Source: CAD feature listing. Evaluate the final solid. Frame: model axes, mm. Give positions to 0.01 mm unless a question says otherwise; leave off trailing zeros. Order: outer loops, then holes, each group sorted by start corner. A loop starts at its lowest first (then second) coordinate and runs counter-clockwise, first axis right, second up.
from build123d import *

# Parameters (mm, degrees)
F1_DEPTH = 0.8
F3_DEPTH = 25


# Not quite as in the source:
# - a feature names something its author has since deleted; it is built from what else it names


with BuildPart() as f1:
    # F0 (on Front) → F1 (new body, symmetric)
    with BuildSketch(Plane.XZ):
        Polygon((609, -150), (609, 150), (-609, 150), (-609, -150), (-98.2216194272, -150), (-98.2216194272, -80), (101.7783805728, -80), (101.7783805728, -150), align=None)
    extrude(amount=F1_DEPTH, both=True)

    # F2 (on face) → F3 (cut)
    with BuildSketch(Plane.XZ.offset(0.8)):
        with BuildLine():
            Line((-609, 0), (-586.7130714899, 0))
            ThreePointArc((-586.7130714899, 0), (-593.05140569, 16.7836636007), (-609, 25))
            Line((-609, 25), (-609, 0))
        make_face()
        with BuildLine():
            ThreePointArc((-460, 0), (-435, -25), (-410, 0))
            Line((-410, 0), (-435, 0))
            Line((-435, 0), (-460, 0))
        make_face()
        with BuildLine():
            Line((-435, 0), (-410, 0))
            ThreePointArc((-410, 0), (-435, 25), (-460, 0))
            Line((-460, 0), (-435, 0))
        make_face()
        with BuildLine():
            ThreePointArc((-286, 0), (-261, -25), (-236, 0))
            Line((-236, 0), (-261, 0))
            Line((-261, 0), (-286, 0))
        make_face()
        with BuildLine():
            Line((-261, 0), (-236, 0))
            ThreePointArc((-236, 0), (-261, 25), (-286, 0))
            Line((-286, 0), (-261, 0))
        make_face()
        with BuildLine():
            ThreePointArc((-112, 0), (-87, -25), (-62, 0))
            Line((-62, 0), (-87, 0))
            Line((-87, 0), (-112, 0))
        make_face()
        with BuildLine():
            Line((-87, 0), (-62, 0))
            ThreePointArc((-62, 0), (-87, 25), (-112, 0))
            Line((-112, 0), (-87, 0))
        make_face()
        with BuildLine():
            ThreePointArc((112, 0), (87, 25), (62, 0))
            Line((62, 0), (87, 0))
            Line((87, 0), (112, 0))
        make_face()
        with BuildLine():
            Line((87, 0), (62, 0))
            ThreePointArc((62, 0), (87, -25), (112, 0))
            Line((112, 0), (87, 0))
        make_face()
        with BuildLine():
            ThreePointArc((286, 0), (261, 25), (236, 0))
            Line((236, 0), (261, 0))
            Line((261, 0), (286, 0))
        make_face()
        with BuildLine():
            Line((261, 0), (236, 0))
            ThreePointArc((236, 0), (261, -25), (286, 0))
            Line((286, 0), (261, 0))
        make_face()
        with BuildLine():
            ThreePointArc((460, 0), (435, 25), (410, 0))
            Line((410, 0), (435, 0))
            Line((435, 0), (460, 0))
        make_face()
        with BuildLine():
            Line((435, 0), (410, 0))
            ThreePointArc((410, 0), (435, -25), (460, 0))
            Line((460, 0), (435, 0))
        make_face()
        with BuildLine():
            ThreePointArc((-609, -24.7047928188), (-593.1499526355, -16.5983450419), (-586.7130714899, 0))
            Line((-586.7130714899, 0), (-609, 0))
            Line((-609, 0), (-609, -24.7047928188))
        make_face()
        with BuildLine():
            ThreePointArc((609, 25), (591.3223304703, 17.6776695297), (584, 0))
            Line((584, 0), (609, 0))
            Line((609, 0), (609, 25))
        make_face()
        with BuildLine():
            Line((609, 0), (584, 0))
            ThreePointArc((584, 0), (591.3223304703, -17.6776695297), (609, -25))
            Line((609, -25), (609, 0))
        make_face()
        with BuildLine():
            ThreePointArc((-532, 0), (-522, -10), (-512, 0))
            Line((-512, 0), (-532, 0))
        make_face()
        with BuildLine():
            Line((-532, 0), (-512, 0))
            ThreePointArc((-512, 0), (-522, 10), (-532, 0))
        make_face()
        with BuildLine():
            ThreePointArc((-358, 0), (-348, -10), (-338, 0))
            Line((-338, 0), (-358, 0))
        make_face()
        with BuildLine():
            Line((-358, 0), (-338, 0))
            ThreePointArc((-338, 0), (-348, 10), (-358, 0))
        make_face()
        with BuildLine():
            ThreePointArc((-184, 0), (-174, -10), (-164, 0))
            Line((-164, 0), (-184, 0))
        make_face()
        with BuildLine():
            Line((-184, 0), (-164, 0))
            ThreePointArc((-164, 0), (-174, 10), (-184, 0))
        make_face()
        with BuildLine():
            Line((0, 0), (-10, 0))
            ThreePointArc((-10, 0), (0, -10), (10, 0))
            Line((10, 0), (0, 0))
        make_face()
        with BuildLine():
            ThreePointArc((10, 0), (0, 10), (-10, 0))
            Line((-10, 0), (0, 0))
            Line((0, 0), (10, 0))
        make_face()
        with BuildLine():
            ThreePointArc((184, 0), (174, 10), (164, 0))
            Line((164, 0), (184, 0))
        make_face()
        with BuildLine():
            Line((184, 0), (164, 0))
            ThreePointArc((164, 0), (174, -10), (184, 0))
        make_face()
        with BuildLine():
            ThreePointArc((358, 0), (348, 10), (338, 0))
            Line((338, 0), (358, 0))
        make_face()
        with BuildLine():
            Line((358, 0), (338, 0))
            ThreePointArc((338, 0), (348, -10), (358, 0))
        make_face()
        with BuildLine():
            ThreePointArc((532, 0), (522, 10), (512, 0))
            Line((512, 0), (532, 0))
        make_face()
        with BuildLine():
            Line((532, 0), (512, 0))
            ThreePointArc((512, 0), (522, -10), (532, 0))
        make_face()
    extrude(amount=-F3_DEPTH, mode=Mode.SUBTRACT)


solid = f1.part
(1) Section A-A, the plane x = 87. Return loops of the section in (y, z).
(2) Line query: line 1 along X through (y, z) = (-0.5, -123.5); line 2 along Z through (x, y) = (0, 0.4); line 3 along Z through (x, y) = (435, 0.1). Output: solid intervals per line, ascending.
(3) Draft query along Z for faces 1 (the flat face through (-9, -0.8, 35)), 2 (the cylindrical face through (-164.763, -0.011, -3.83)). Return one class per face: +Z half, -Z half, draft (parallel to the pull), parting line (faces both ways), or undercut.
(4) Pin query (flat end, axial travel): pin 1 Ø0.8 at (x, y) = (-43.5, -0.5) entering from -Z. Return the tip coordinate at first contact, or that it passes through.
(5) Section C-C, the plane y = 0.45. Count the separate pieces of the cut face and the enclosed holes in it, plus the area to 3 significant figures.
(6) Section B-B, the plane z = -127.5. Return loops of the section in (x, y), plus the area to 3 significant figures.
Checks:
1. outline: (-0.8, -80) - (0.8, -80) - (0.8, -25) - (-0.8, -25) - close; (-0.8, 25) - (0.8, 25) - (0.8, 150) - (-0.8, 150) - close
2. line 1: x = -609 to -98.22, 101.78 to 609
2. line 2: z = -80 to -10, 10 to 150
2. line 3: z = -150 to -25, 25 to 150
3. face 1: draft
3. face 2: undercut
4. pin 1: stops at z = -80
5. separate pieces: 1
5. enclosed holes: 13
5. area: 336,000 mm2
6. outline: (-609, -0.8) - (-98.22, -0.8) - (-98.22, 0.8) - (-609, 0.8) - close; (101.78, -0.8) - (609, -0.8) - (609, 0.8) - (101.78, 0.8) - close
6. area: 1,630 mm2
